Here's how the part is built. I have some questions about the finished solid (model axes, mm). Round coordinates to 2 decimals unless told otherwise and drop trailing zeros. Write each loop counter-clockwise with the first axis right and the second up, starting at its lowest first coordinate (ties: lowest second). Pieces come first, ordered by that corner, then holes. Notation, with made-up numbers: (44.25, -22) -> (89.25, -22) arc R18 ccw to (89.25, -15) -> close; hole circle Ø3 at (64, 47). An arc over 180 degrees is marked (long way). Answer as CSV lines item,"result".
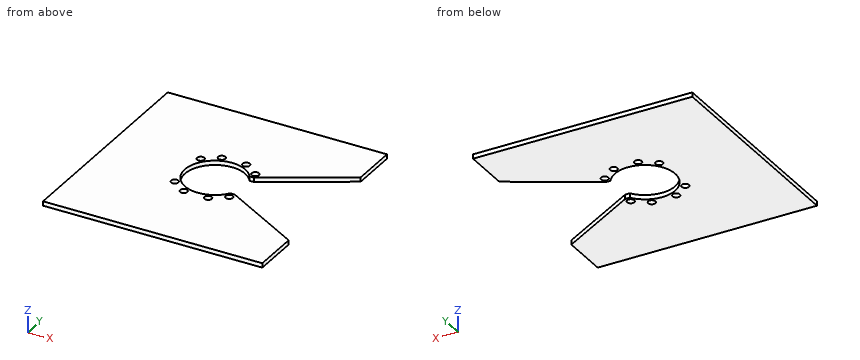
from build123d import *

# Parameters (mm, degrees)
F0_R     = 16.5
F1_DEPTH = 20


with BuildPart() as f1:
    # F0 (on Top) → F1 (new body)
    with BuildSketch(Plane.XY):
        with BuildLine():
            ThreePointArc((113.578167, -77.5), (-137.5, 0), (113.578167, 77.5))
            Line((113.578167, 77.5), (134.233938, 77.5))
            Line((134.233938, 77.5), (500, 288.675135))
            Line((500, 288.675135), (500, 500))
            Line((500, 500), (-500, 500))
            Line((-500, 500), (-500, -500))
            Line((-500, -500), (500, -500))
            Line((500, -500), (500, -288.675135))
            Line((500, -288.675135), (134.233938, -77.5))
            Line((134.233938, -77.5), (113.578167, -77.5))
        make_face()
        with Locations((-55.578273, -152.700051)):
            Circle(F0_R, mode=Mode.SUBTRACT)
        with Locations((-124.482222, -104.452987)):
            Circle(F0_R, mode=Mode.SUBTRACT)
        with Locations((55.578273, -152.700051)):
            Circle(F0_R, mode=Mode.SUBTRACT)
        with Locations((124.482222, -104.452987)):
            Circle(F0_R, mode=Mode.SUBTRACT)
        with Locations((-124.482222, 104.452987)):
            Circle(F0_R, mode=Mode.SUBTRACT)
        with Locations((-55.578273, 152.700051)):
            Circle(F0_R, mode=Mode.SUBTRACT)
        with Locations((124.482222, 104.452987)):
            Circle(F0_R, mode=Mode.SUBTRACT)
        with Locations((55.578273, 152.700051)):
            Circle(F0_R, mode=Mode.SUBTRACT)
    extrude(amount=F1_DEPTH)


solid = f1.part
Item 1: Suppose I cut it at B-B, the plane z = 16. State how many separate pieces and enclosed holes the cut face has, then the cut area to 3 significant figures.
Results found:
separate pieces,"1"
enclosed holes,"8"
area,"799,000 mm²"
Item 2: Suppose I cut it at A-A, the plane x = 0. List the corners of the cut face in (y, z) for me, then the cut area to 3 significant figures.
Results found:
outline,"(-500, 0) -> (-137.5, 0) -> (-137.5, 20) -> (-500, 20) -> close; (137.5, 0) -> (500, 0) -> (500, 20) -> (137.5, 20) -> close"
area,"14,500 mm²"
Item 3: Suppose I cut it at C-C, the plane x = 279. List the corners of the cut face in (y, z) for me, then the cut area to 3 significant figures.
Results found:
outline,"(-500, 0) -> (-161.08, 0) -> (-161.08, 20) -> (-500, 20) -> close; (161.08, 0) -> (500, 0) -> (500, 20) -> (161.08, 20) -> close"
area,"13,600 mm²"
Item 4: I need wall thicknesses on L1, parallel to Y at x = 0, z = 6.25; L2, parallel to X at y = 159.5, z = 15; L3, parallel to Y at x = 152, z = 19. Which ranges of each line are inside material? Lowest first, please.
Results found:
L1,"y = -500 to -137.5, 137.5 to 500"
L2,"x = -500 to -70.61, -40.54 to 40.54, 70.61 to 276.26"
L3,"y = -500 to -87.76, 87.76 to 500"
Item 5: Will this pin go through, and if not, where does the flat tip stop? pin 1 (12 mm diameter, centred on y = 275.5, z = 16.5, fed in from +X).
Results found:
pin 1,"stops at x = 487.57"
Item 6: Suppose I cut it at D-D, the plane y = 0. List the corners of the cut face in (x, z) for me.
Results found:
outline,"(-500, 0) -> (-137.5, 0) -> (-137.5, 20) -> (-500, 20) -> close"
